Can you work these out from the model? Positions are in its coordinate system, mm. Face numbers are marked on the shaded views. Round coordinates to 2 decimals unless told otherwise and drop trailing zeros. Order: outer loops, then holes, each group sorted by start corner. A loop starts at its lowest first (then second) coordinate and runs counter-clockwise, first axis right, second up. Notation, with made-up numbers: M -31.5,-2 L -15.5,-2 A32 ccw -15.5,37 Z; hole C -40,40 d10. An arc over 180 degrees is marked long. One line per question, with ' | ' between items.
```python
from build123d import *

# Parameters (mm, degrees)
F3_W     = 22
F3_H     = 22
F4_DEPTH = 5.5
F5_R     = 3
F6_R     = 5.5
F7_DEPTH = 5.5
F7_TAPER = -10


with BuildPart() as f4:
    # F3 (on Top) → F4 (new body)
    with BuildSketch(Plane.XY):
        Rectangle(F3_W, F3_H)
    extrude(amount=F4_DEPTH)

    # F5
    f5_edges = [f4.edges().sort_by_distance(p)[0] for p in [
        (11, -11, 2.75),
        (11, 11, 2.75),
        (-11, 11, 2.75),
        (-11, -11, 2.75),
    ]]
    fillet(f5_edges, radius=F5_R)

    # F6 (on face) → F7 (cut, through all)
    with BuildSketch(Plane(origin=(0, 0, 0), x_dir=(1, 0, 0), z_dir=(0, 0, -1))):
        Circle(F6_R)
    extrude(amount=-F7_DEPTH, taper=F7_TAPER, mode=Mode.SUBTRACT)


solid = f4.part
```
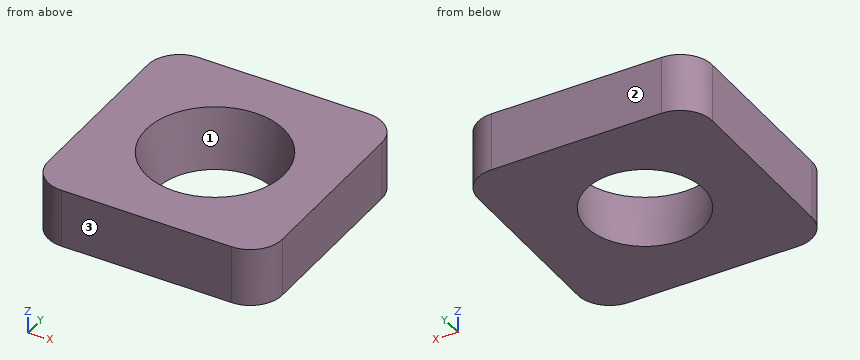
(1) If we section it at B-B on z = 2: Please give me the cut outline in (x, y), plus the area to 3 significant figures.
Final values:
outline: M -11,-8 A3 ccw -8,-11 L 8,-11 A3 ccw 11,-8 L 11,8 A3 ccw 8,11 L -8,11 A3 ccw -11,8 Z; hole C 0,0 d11.71 | area: 369 mm^2
(2) If we section it at D-D on x = -9: Please give me the cut outline in (y, z), plus the area to 3 significant figures.
Final values:
outline: M -10.83,0 L 10.83,0 L 10.83,5.5 L -10.83,5.5 Z | area: 119 mm^2
(3) If we section it at C-C on z = 4: Please give me the cut outline in (x, y).
Final values:
outline: M -11,-8 A3 ccw -8,-11 L 8,-11 A3 ccw 11,-8 L 11,8 A3 ccw 8,11 L -8,11 A3 ccw -11,8 Z; hole C 0,0 d12.41
(4) Thinking about a two-plate mould opening in Y: for the marked faces 1, 2 and 3, which applies, released by +Y, released by -Y, zero draft, split by the parting line, or undercut?
Final values:
face 1: undercut | face 2: released by +Y | face 3: released by -Y
(5) Please list where these lines run through material, in increasing order: probe 1 along X at (y, z) = (3.75, 1.15); probe 2 along Y at (x, z) = (-3.25, 3.3); probe 3 along X at (y, z) = (-5, 0.9). Write a range as [from, to].
Final values:
probe 1: [-11, -4.3], [4.3, 11] | probe 2: [-11, -5.14], [5.14, 11] | probe 3: [-11, -2.65], [2.65, 11]
(6) If we section it at A-A on x = 0: Please give me the cut outline in (y, z).
Final values:
outline: M -11,0 L -5.5,0 L -6.47,5.5 L -11,5.5 Z; M 5.5,0 L 11,0 L 11,5.5 L 6.47,5.5 Z
